from build123d import *

# Parameters (mm, degrees)
SKETCH5_R = 1


with BuildPart() as part:
    # Sweep1: sweep along a curve in space
    with BuildLine() as sweep1_path:
        Line((13, 0, 0), (0, 0, 0))
        Line((13, 0, -20), (13, 0, 0))
        Line((23, 0, -20), (13, 0, -20))
        Line((23, 0, 0), (23, 0, -20))
        Line((53, 0, 0), (23, 0, 0))
        Line((53, 0, 0), (53, 15.636629649, -12.469796037))
        Line((53, 15.636629649, -12.469796037), (63, 15.636629649, -12.469796037))
        Line((63, 15.636629649, -12.469796037), (63, 0, 0))
        Line((63, 0, 0), (93, 0, 0))
        Line((93, 0, 0), (93, 19.498558244, 4.450418679))
        Line((93, 19.498558244, 4.450418679), (103, 19.498558244, 4.450418679))
        Line((103, 19.498558244, 4.450418679), (103, 0, 0))
        Line((103, 0, 0), (133, 0, 0))
        Line((133, 0, 0), (133, 8.677674782, 18.019377358))
        Line((133, 8.677674782, 18.019377358), (143, 8.677674782, 18.019377358))
        Line((143, 8.677674782, 18.019377358), (143, 0, 0))
        Line((143, 0, 0), (173, 0, 0))
        Line((173, 0, 0), (173, -8.677674782, 18.019377358))
        Line((173, -8.677674782, 18.019377358), (183, -8.677674782, 18.019377358))
        Line((183, -8.677674782, 18.019377358), (183, 0, 0))
        Line((183, 0, 0), (213, 0, 0))
        Line((213, 0, 0), (213, -19.498558244, 4.450418679))
        Line((213, -19.498558244, 4.450418679), (223, -19.498558244, 4.450418679))
        Line((223, -19.498558244, 4.450418679), (223, 0, 0))
        Line((223, 0, 0), (253, 0, 0))
        Line((253, 0, 0), (253, -15.636629649, -12.469796037))
        Line((253, -15.636629649, -12.469796037), (263, -15.636629649, -12.469796037))
        Line((263, -15.636629649, -12.469796037), (263, 0, 0))
        Line((263, 0, 0), (300, 0, 0))
    # Sketch5 → Sweep1 (sweep)
    with BuildSketch(Plane(origin=(0, 0, 0), x_dir=(0, 0, -1), z_dir=(1, 0, 0))):
        Circle(SKETCH5_R)
    sweep(path=sweep1_path.line, transition=Transition.RIGHT)


solid = part.part
Check sheet for the modelled part. Datum: model origin and axes. Units: mm. Round coordinates to 2 decimals unless told otherwise and drop trailing zeros. Loops run counter-clockwise (first coordinate to the right, second up) from the corner with the lowest first, then second, coordinate; pieces in that order, holes last. Notation, with made-up numbers: (-32.5, 78.5) -> (19.5, 78.5) arc R32 ccw to (19.5, 112.5) -> close; hole circle Ø11 at (-33, 4.25). An arc over 180 degrees is marked (long way). Put each result on its own line as item: value. Start each with the question number.
1. Scan lines: probe 1 along Y at (x, z) = (156, 0); probe 2 along X at (y, z) = (-6, 0.5); probe 3 along X at (y, z) = (-2, 5). Record each from-to range of solid material in increasing order.
2. Section check B-B (z = -6). Give the number of separate pieces and of enclosed holes in the cut face, plus the area to 3 significant figures.
3. Section check A-A (x = 153). Enter the section's corners in (y, z), plus the area to 3 significant figures.
4. Gauge pin test, flat ends, axial feed: pin 1 (4 mm diameter, centred on y = 1.5, z = 3.5, fed in from -X); pin 2 (8 mm diameter, centred on x = 233, z = 8, fed in from -Y); pin 3 (6 mm diameter, centred on x = 61.5, z = -6.5, fed in from -Y); pin 4 (5 mm diameter, centred on x = 235.5, z = 1, fed in from -Y). Record the tip position at first contact, or that the pin passes through.
Findings:
1. probe 1: y = -1 to 1
1. probe 2: x = 212.47 to 213.53, 222.47 to 223.53
1. probe 3: x = 172.07 to 173.93, 182.07 to 183.93
2. separate pieces: 6
2. enclosed holes: 0
2. area: 26.4 mm^2
3. outline: circle Ø2 at (0, 0)
3. area: 3.14 mm^2
4. pin 1: stops at x = 132
4. pin 2: passes through
4. pin 3: stops at y = 3.17
4. pin 4: stops at y = -1
